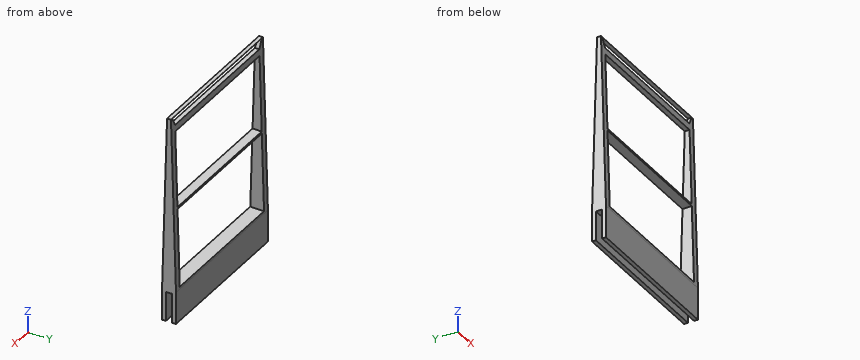
```python
from build123d import *

# Parameters (mm, degrees)
F1_DEPTH = 40
F2_W     = 73.3336731791
F2_H     = 38.809017675
F2_H_2   = 1
F3_DEPTH = 7.5685053212


# Not quite as in the source:
# - a feature names something its author has since deleted; it is built from what else it names


with BuildPart() as f1:
    # F0 (on Right) → F1 (new body, symmetric)
    with BuildSketch(Plane.YZ):
        Polygon((-1.55, -15), (-1.55, 0), (1.55, 0), (1.55, -15), (3.55, -15), (3.55, 1.359729562), (1, 90), (-1, 90), (-3.55, 1.359729562), (-3.55, 0), (-3.55, -15), align=None)
    extrude(amount=F1_DEPTH, both=True)

    # F2 (on face) → F3 (cut, through all)
    with BuildSketch(Plane(origin=(0, -3.5861487682, 0.1031661943), x_dir=(1, 0, 0), z_dir=(0, -0.9995864588, 0.028756066))):
        Polygon((36.6668365896, 85.5283662677), (39.0464413553, 89.9340252282), (-39.0464413553, 89.9340252282), (-36.6668365896, 85.5283662677), align=None)
        with Locations((0, 62.7911531245)):
            Rectangle(F2_W, F2_H)
        with Locations((0, 41.886644287)):
            Rectangle(F2_W, F2_H_2)
        with Locations((0, 21.9821354495)):
            Rectangle(F2_W, F2_H)
    extrude(amount=-F3_DEPTH, mode=Mode.SUBTRACT)


solid = f1.part
```
CAD build for the part. Positions are in the model's coordinates, mm. Round coordinates to 2 decimals unless told otherwise and drop trailing zeros. Order: outer loops, then holes, each group sorted by start corner. A loop starts at its lowest first (then second) coordinate and runs counter-clockwise, first axis right, second up. Notation, with made-up numbers: (-10, -3.5) - (36, -3.5) arc R14 ccw to (36, 18.5) - close; hole circle Ø9 at (-14.5, -11.75). An arc over 180 degrees is marked (long way). Answer in a Markdown table with one row per item. Add a question column.
(1) Band-saw the part on C-C on z = 35.5. List the corners of the cut face in (x, y).
(2) Band-saw the part on A-A on x = 13. List the corners of the cut face in (y, z).
(3) Probe L1, parallel to X at y = 0.5, z = 59.5; L2, parallel to Z at x = -21.5, y = 3; L3, parallel to Z at x = 24, y = -3 (3 decimals). List the from-to ranges inside material, lowest first. Write a range as [from, to].
(4) Band-saw the part on B-B on z = 72.5. List the corners of the cut face in (x, y).
Data:
| question | item | result |
|---|---|---|
| 1 | outline | (-40, -2.57) - (-36.67, -2.57) - (-36.67, 2.57) - (-40, 2.57) - close; (36.67, -2.57) - (40, -2.57) - (40, 2.57) - (36.67, 2.57) - close |
| 2 | outline | (-3.55, -15) - (-1.55, -15) - (-1.55, 0) - (1.55, 0) - (1.55, -15) - (3.55, -15) - (3.55, 1.36) - (3.52, 2.48) - (-3.51, 2.68) - (-3.55, 1.36) - close; (-2.37, 42.47) - (2.37, 42.34) - (2.34, 43.34) - (-2.34, 43.47) - close; (-1.22, 82.26) - (1.22, 82.19) - (1.13, 85.53) - (-1.13, 85.6) - close; (-1, 90) - (1, 89.94) - (1, 90) - close |
| 3 | L1 | x = [-40, -36.67], [36.67, 40] |
| 3 | L2 | z = [-15, 2.49] |
| 3 | L3 | z = [-15, 2.665] |
| 4 | outline | (-40, -1.5) - (-36.67, -1.5) - (-36.67, 1.5) - (-40, 1.5) - close; (36.67, -1.5) - (40, -1.5) - (40, 1.5) - (36.67, 1.5) - close |
